Could you check a few things on this model? Use its own coordinates, in mm. A direction names the side the tool comes from. Round coordinates to 2 decimals unless told otherwise and drop trailing zeros. Loops run counter-clockwise (first coordinate to the right, second up) from the corner with the lowest first, then second, coordinate; pieces in that order, holes last. Notation, with made-up numbers: M 83,45.5 L 126,45.5 A19 ccw 126,52.5 Z; hole C -16,0.25 d4. An arc over 180 degrees is marked long. One line per item, written item: value. Start each with the question number.
Q1. I'm going to push flat-ended pins straight in: pin 1 Ø3 at (y, z) = (-147, -25) entering from -X; pin 2 Ø3 at (x, y) = (13, -146) entering from -Z; pin 3 Ø2 at (x, y) = (-2, -144) entering from +Z. Where does each tip first touch, or does it pass through?
Q2. Which directions (+Z, -Z, +X, -X, +Y, -Y) give clear straight access to the entire face, cutting with the end or side of a thin tool? Please do faces 4 (the face through (-28.956, -146, -7)), 5 (the face through (-22.606, -146, -216)), 6 (the face through (13, -146, -182.562)), 7 (the face through (13, -146, -209.55)).
Q3. Imagine slicing it at B-B (z = -164.5). Please give me the cut outline in (x, y).
Q4. Thinking about a two-plate mould opening in X: for faces 1 (the face through (9.652, -146, 3)), 2 (the face through (9.652, -146, -108)), 3 (the face through (-26, -146, -87.312)), which applies, released by +X, released by -X, zero draft, split by the parting line, or undercut?
Q5. Imagine slicing it at A-A (x = -2). Please give me the cut outline in (y, z), then the cut area to 3 significant figures.
Q6. Please list where these lines run through material, in increasing order: line 1 along Z through (x, y) = (-8.5, -147.75); line 2 along X through (y, z) = (-143.5, -27.5).
from build123d import *

# Parameters (mm, degrees)
SKETCH1_W           = 44.958
SKETCH1_H           = 304.8
BOSS_EXTRUDE1_DEPTH = 6.35
SKETCH2_W           = 6.35
SKETCH2_H           = 101.6
BOSS_EXTRUDE2_DEPTH = 6.35
SKETCH3_W           = 222.25
SKETCH3_H           = 6.35
BOSS_EXTRUDE3_DEPTH = 38.608
SKETCH7_W           = 333.372738736
SKETCH7_H           = 323.725005723
CUT_EXTRUDE1_DEPTH  = 45.958
SKETCH4_W           = 6.35
SKETCH4_H           = 12.7
CUT_EXTRUDE2_DEPTH  = 6.35
SKETCH8_W           = 6.477
SKETCH8_H           = 6.35
SKETCH8_W_2         = 19.431
CUT_EXTRUDE4_DEPTH  = 7.35


with BuildPart() as part:
    # Sketch1 → Boss-Extrude1 (new body)
    with BuildSketch(Plane.XY):
        with Locations((-6.477, 3.048)):
            Rectangle(SKETCH1_W, SKETCH1_H)
        with BuildLine():
            Line((-3.302, 133.858), (-3.302, -143.002))
            Line((-3.302, -143.002), (3.302, -143.002))
            Line((3.302, -143.002), (3.302, 143.002))
            Line((3.302, 143.002), (-16.256, 143.002))
            Line((-16.256, 143.002), (-16.256, 136.398))
            Line((-16.256, 136.398), (-5.842, 136.398))
            ThreePointArc((-5.842, 136.398), (-4.045948776, 135.654051224), (-3.302, 133.858))
        make_face(mode=Mode.SUBTRACT)
    extrude(amount=BOSS_EXTRUDE1_DEPTH)

    # Sketch2 → Boss-Extrude2 (add)
    with BuildSketch(Plane(origin=(16.002, 0, 0), x_dir=(0, 0, -1), z_dir=(1, 0, 0))):
        Polygon((222.25, -60.452), (222.25, -47.752), (0, -47.752), (0, -149.352), (222.25, -149.352), (222.25, -136.652), (228.6, -136.652), (228.6, -119.718666667), (222.25, -119.718666667), (222.25, -107.018666667), (228.6, -107.018666667), (228.6, -90.085333333), (222.25, -90.085333333), (222.25, -77.385333333), (228.6, -77.385333333), (228.6, -60.452), align=None)
        with BuildLine():
            ThreePointArc((11.4, -116.592), (9.9, -118.092), (8.4, -116.592))
            Line((8.4, -116.592), (8.4, -111.512))
            ThreePointArc((8.4, -111.512), (9.9, -110.012), (11.4, -111.512))
            Line((11.4, -111.512), (11.4, -116.592))
        make_face(mode=Mode.SUBTRACT)
        with BuildLine():
            Line((42.4, -111.512), (42.4, -116.592))
            ThreePointArc((42.4, -116.592), (40.9, -118.092), (39.4, -116.592))
            Line((39.4, -116.592), (39.4, -111.512))
            ThreePointArc((39.4, -111.512), (40.9, -110.012), (42.4, -111.512))
        make_face(mode=Mode.SUBTRACT)
        with BuildLine():
            ThreePointArc((36.4, -101.092), (25.4, -112.092), (14.4, -101.092))
            Line((14.4, -101.092), (14.4, -96.012))
            ThreePointArc((14.4, -96.012), (25.4, -85.012), (36.4, -96.012))
            Line((36.4, -96.012), (36.4, -101.092))
        make_face(mode=Mode.SUBTRACT)
        with BuildLine():
            ThreePointArc((11.4, -85.592), (9.9, -87.092), (8.4, -85.592))
            Line((8.4, -85.592), (8.4, -80.512))
            ThreePointArc((8.4, -80.512), (9.9, -79.012), (11.4, -80.512))
            Line((11.4, -80.512), (11.4, -85.592))
        make_face(mode=Mode.SUBTRACT)
        with BuildLine():
            ThreePointArc((42.4, -85.592), (40.9, -87.092), (39.4, -85.592))
            Line((39.4, -85.592), (39.4, -80.512))
            ThreePointArc((39.4, -80.512), (40.9, -79.012), (42.4, -80.512))
            Line((42.4, -80.512), (42.4, -85.592))
        make_face(mode=Mode.SUBTRACT)
        with Locations((-3.175, -98.552)):
            Rectangle(SKETCH2_W, SKETCH2_H)
    extrude(amount=-BOSS_EXTRUDE2_DEPTH)

    # Sketch3 → Boss-Extrude3 (add)
    with BuildSketch(Plane.ZY.offset(-9.652)):
        with Locations((-111.125, -146.177)):
            Rectangle(SKETCH3_W, SKETCH3_H)
    extrude(amount=BOSS_EXTRUDE3_DEPTH)

    # Sketch7 → Cut-Extrude1 (cut, through all)
    with BuildSketch(Plane(origin=(16.002, 0, 0), x_dir=(0, 0, -1), z_dir=(1, 0, 0))):
        with Locations((160.336369368, 18.860502861)):
            Rectangle(SKETCH7_W, SKETCH7_H)
    extrude(amount=-CUT_EXTRUDE1_DEPTH, mode=Mode.SUBTRACT)

    # Sketch4 → Cut-Extrude2 (cut)
    with BuildSketch(Plane.XZ.offset(149.352)):
        with Locations((12.827, -26.9875)):
            Rectangle(SKETCH4_W, SKETCH4_H)
        with Locations((-25.781, -26.9875)):
            Rectangle(SKETCH4_W, SKETCH4_H)
        with Locations((-25.781, -53.975)):
            Rectangle(SKETCH4_W, SKETCH4_H)
        with Locations((-25.781, -80.9625)):
            Rectangle(SKETCH4_W, SKETCH4_H)
        with Locations((-25.781, -107.95)):
            Rectangle(SKETCH4_W, SKETCH4_H)
        with Locations((-25.781, -134.9375)):
            Rectangle(SKETCH4_W, SKETCH4_H)
        with Locations((-25.781, -161.925)):
            Rectangle(SKETCH4_W, SKETCH4_H)
        with Locations((-25.781, -188.9125)):
            Rectangle(SKETCH4_W, SKETCH4_H)
        with Locations((-25.781, -215.9)):
            Rectangle(SKETCH4_W, SKETCH4_H)
        with Locations((12.827, -215.9)):
            Rectangle(SKETCH4_W, SKETCH4_H)
        with Locations((12.827, -161.925)):
            Rectangle(SKETCH4_W, SKETCH4_H)
        with Locations((12.827, -134.9375)):
            Rectangle(SKETCH4_W, SKETCH4_H)
        with Locations((12.827, -107.95)):
            Rectangle(SKETCH4_W, SKETCH4_H)
        with Locations((12.827, -80.9625)):
            Rectangle(SKETCH4_W, SKETCH4_H)
        with Locations((12.827, -53.975)):
            Rectangle(SKETCH4_W, SKETCH4_H)
        with Locations((12.827, -188.9125)):
            Rectangle(SKETCH4_W, SKETCH4_H)
    extrude(amount=-CUT_EXTRUDE2_DEPTH, mode=Mode.SUBTRACT)

    # Sketch8 → Cut-Extrude4 (cut, through all)
    with BuildSketch(Plane.XZ.offset(149.352)):
        with Locations((-19.3675, 3.175)):
            Rectangle(SKETCH8_W, SKETCH8_H)
        with Locations((-0.0635, 3.175)):
            Rectangle(SKETCH8_W_2, SKETCH8_H)
    extrude(amount=-CUT_EXTRUDE4_DEPTH, mode=Mode.SUBTRACT)


solid = part.part
Report:
1. pin 1: stops at x = -22.61
1. pin 2: stops at z = -209.55
1. pin 3: stops at z = 0
2. face 4: +Z, -Z, -X, +Y, -Y
2. face 5: -Z, -X, +Y, -Y
2. face 6: +X, +Y, -Y
2. face 7: -Z, +X, +Y, -Y
3. outline: M -22.61,-149.35 L 9.65,-149.35 L 9.65,-143 L -22.61,-143 Z
4. face 1: undercut
4. face 2: released by +X
4. face 3: zero draft
5. outline: M -149.35,-222.25 L -143,-222.25 L -143,0 L -149.35,0 Z
5. area: 1,410 mm²
6. line 1: z = -222.25 to 0
6. line 2: x = -22.61 to 9.65
